Work out the finished part from the listing and answer in its coordinate system (mm). A direction names the side the tool comes from. Round coordinates to 2 decimals unless told otherwise and drop trailing zeros. Write each loop counter-clockwise with the first axis right and the second up, starting at its lowest first coordinate (ties: lowest second). Pieces come first, ordered by that corner, then holes. Notation, with made-up numbers: M 2,56.25 L 46,56.25 A18 cw 46,67.25 Z; hole C -32,-25 d7. An arc over 180 degrees is marked long. Answer in a Markdown table with one row per item.
```python
from build123d import *

# Parameters (mm, degrees)
SCHIZZO1_R                        = 5
ESTRUSIONE_ESTRUSIONE1_DEPTH      = 12
ESTRUSIONE_ESTRUSIONE2_DEPTH      = 20
ESTRUSIONE_ESTRUSIONE2_DEPTH_BACK = 5
SCHIZZO3_W                        = 5
SCHIZZO3_H                        = 20
RACCORDO1_R                       = 20
RACCORDO2_R                       = 10
RACCORDO3_R                       = 10
TAGLIO_ESTRUSIONE1_DEPTH          = 122.866986916
TAGLIO_ESTRUSIONE1_DEPTH_BACK     = 122.866986916
SCHIZZO4_R                        = 5


# Some blends are built 0.0001 mm under size
with BuildPart() as part:
    # Schizzo1 → Estrusione-Estrusione1 (new body)
    with BuildSketch(Plane.XY):
        with BuildLine():
            Line((0, 10), (100, 10))
            Line((100, 10), (100, -10))
            Line((100, -10), (0, -10))
            ThreePointArc((0, -10), (-10, 0), (0, 10))
        make_face()
        Circle(SCHIZZO1_R, mode=Mode.SUBTRACT)
    extrude(amount=ESTRUSIONE_ESTRUSIONE1_DEPTH)

    # Schizzo3 → Estrusione-Estrusione2 (add, two sides: drawn at the far end of the back side and taken through both)
    with BuildSketch(Plane(origin=(100, 0, 0), x_dir=(0, 0, -1), z_dir=(1, 0, 0)).offset(-ESTRUSIONE_ESTRUSIONE2_DEPTH_BACK)):
        with Locations((-12.875, 0)):
            Rectangle(SCHIZZO3_W, SCHIZZO3_H)
        with Locations((0.875, 0)):
            Rectangle(SCHIZZO3_W, SCHIZZO3_H)
    extrude(amount=ESTRUSIONE_ESTRUSIONE2_DEPTH + ESTRUSIONE_ESTRUSIONE2_DEPTH_BACK)

    # Raccordo1
    # the kernel refuses this fillet: 20 mm, written as the material it adds along each edge
    with BuildSketch(Plane(origin=(95, 10, 12), x_dir=(-1, 0, 0), z_dir=(0, -1, 0)), Plane(origin=(95, -10, 0), x_dir=(-1, 0, 0), z_dir=(0, 1, 0))) as raccordo1_piece_1:
        with BuildLine():
            CenterArc((11.11797531, -20), RACCORDO1_R, 90, 33.772641851)
            Line((0, -3.375), (-0.222359506, -3.0425))
            ThreePointArc((-0.222359506, -3.0425), (-0.4, -1.6875), (-0.4, 0))
            Line((-0.4, 0), (0, 0.4))
            Line((0, 0.4), (11.11797531, 0.4))
            Line((11.11797531, 0.4), (11.11797531, 0))
        make_face()
    extrude(amount=20)

    # Raccordo2
    raccordo2_edges = [part.edges().sort_by_distance(p)[0] for p in [
        (95, 0, -3.375),
        (95, 0, 15.375),
    ]]
    fillet(raccordo2_edges, radius=RACCORDO2_R)

    # Raccordo3
    raccordo3_edges = [part.edges().sort_by_distance(p)[0] for p in [
        (120, -10, 12.875),
        (120, 10, 12.875),
        (120, -10, -0.875),
        (120, 10, -0.875),
    ]]
    fillet(raccordo3_edges, radius=RACCORDO3_R - 0.0001)  # a hair under: the kernel refuses the full size

    # Schizzo4 → Taglio-Estrusione1 (cut, two sides: drawn at the far end of the back side and taken through both)
    with BuildSketch(Plane(origin=(0, 0, -3.375), x_dir=(-1, 0, 0), z_dir=(0, 0, -1)).offset(-TAGLIO_ESTRUSIONE1_DEPTH_BACK)):
        with Locations(Location((-110, 0, 0), (0, 0, 90))):
            Circle(SCHIZZO4_R)
    extrude(amount=TAGLIO_ESTRUSIONE1_DEPTH + TAGLIO_ESTRUSIONE1_DEPTH_BACK, mode=Mode.SUBTRACT)


solid = part.part
```
1. Consider line 1 along Y through (x, z) = (110, -0.8); line 2 along Z through (x, y) = (104, 3.75) (3 decimals); line 3 along X through (y, z) = (-2.25, 0.5). Determine where each line is inside the solid, lowest interval first. Write a range as from..to.
Calculated:
| item | result |
|---|---|
| line 1 | y = -10..-5, 5..10 |
| line 2 | z = -3.375..1.625, 10.375..15.375 |
| line 3 | x = -9.74..-4.47, 4.47..105.53, 114.47..119.74 |
2. The part is cut by section B-B (x = 78). Determine the outline of the cut face in (y, z), plus the area to 3 significant figures.
Calculated:
| item | result |
|---|---|
| outline | M -10,0 L 10,0 L 10,12 L -10,12 Z |
| area | 240 mm² |
3. The part is cut by section C-C (y = 7.5). Determine the outline of the cut face in (x, z) (3 decimals), plus the area to 3 significant figures.
Calculated:
| item | result |
|---|---|
| outline | M -6.614,0 L 83.882,0 A20 cw 93.098,-2.25 A10 ccw 97.706,-3.375 L 116.614,-3.375 L 116.614,1.625 L 100,1.625 L 100,10.375 L 116.614,10.375 L 116.614,15.375 L 97.706,15.375 A10 ccw 93.098,14.25 A20 cw 83.882,12 L -6.614,12 Z |
| area | 1,500 mm² |
4. The part is cut by section A-A (y = -7). Determine the outline of the cut face in (x, z) (3 decimals), plus the area to 3 significant figures.
Calculated:
| item | result |
|---|---|
| outline | M -7.141,0 L 83.882,0 A20 cw 93.098,-2.25 A10 ccw 97.706,-3.375 L 117.141,-3.375 L 117.141,1.625 L 100,1.625 L 100,10.375 L 117.141,10.375 L 117.141,15.375 L 97.706,15.375 A10 ccw 93.098,14.25 A20 cw 83.882,12 L -7.141,12 Z |
| area | 1,510 mm² |
5. Given pin 1 (2 mm diameter, centred on y = 6, z = 2, fed in from -X); pin 2 (6 mm diameter, centred on x = 16.5, y = -4, fed in from -Z); pin 3 (6 mm diameter, centred on x = 28, y = -3.5, fed in from +Z); pin 4 (6 mm diameter, centred on x = 0, y = 0, fed in from -Z), each flat-ended and moving along its own axis, determine where each tip first touches the part or whether it passes through.
Calculated:
| item | result |
|---|---|
| pin 1 | stops at x = -8.66 |
| pin 2 | stops at z = 0 |
| pin 3 | stops at z = 12 |
| pin 4 | passes through |
6. A tool of negligible diameter and unlimited length cuts with its end or side. For faces 1 (the cylindrical face through (105.12, -1.08, 12.91)), 2 (the flat face through (38, 0, 12)), 3 (the flat face through (100, 0, 6)), from which of +Z, -Z, +X, -X, +Y, -Y can it reach the whole face along a straight path? Write none if from no direction.
Calculated:
| item | result |
|---|---|
| face 1 | +Z, -Z |
| face 2 | +Z, -X, +Y, -Y |
| face 3 | +X, +Y, -Y |
7. Determine the mould class of faces 4 (the cylindrical face through (-10, 0, 6)), 5 (the flat face through (105, 2, 10.375)), 6 (the flat face through (38, 0, 0)) for opening direction Z: released by +Z, released by -Z, zero draft, split by the parting line, or undercut.
Calculated:
| item | result |
|---|---|
| face 4 | zero draft |
| face 5 | undercut |
| face 6 | released by -Z |
